Verification items for the finished model (mm, model axes). Round coordinates to 2 decimals unless told otherwise and drop trailing zeros. Order: outer loops, then holes, each group sorted by start corner. A loop starts at its lowest first (then second) coordinate and runs counter-clockwise, first axis right, second up. Notation, with made-up numbers: (23, -3) -> (68, -3) arc R14 cw to (68, 19) -> close; hole circle Ø2 at (69.5, 69). An arc over 180 degrees is marked (long way). Put each result on its own line as item: value.
```python
from build123d import *

# Parameters (mm, degrees)
PAD012_DEPTH            = 3
FILLET037_R             = 3.35
SKETCH185_R             = 1.15
POCKET053_DEPTH         = 3
POCKET056_DEPTH         = 5
SKETCH189_W             = 32
SKETCH189_H             = 20
POCKET057_DEPTH         = 1.5
BODY024_PLACEMENT_ANGLE = 149
CLONE_PLACEMENT_ANGLE   = 149


with BuildPart() as part:
    # Sketch184 → Pad012 (new body)
    with BuildSketch(Plane(origin=(0, 0, 0), x_dir=(1, 0, 0), z_dir=(0, 0, -1))):
        Polygon((101.467362, -402.500006), (130.400002, -402.500006), (135.400002, -402.500006), (135.400002, -397.500006), (174.999975, -357.90402), (174.999975, -245), (289.999995, -245), (294.999995, -245), (294.999995, -215), (289.999995, -215), (224.999995, -215), (224.999995, -199.999997), (219.999995, -199.999997), (199.999995, -199.999997), (194.999995, -199.999997), (194.999995, -215.000003), (168.459985, -215.000003), (161.999993, -198.359996), (161.999993, -115.000006), (161.999993, -110.000006), (156.999993, -110.000006), (134.576923, -122.534363), (131.999997, -126.895911), (131.999997, -200.027011), (144.989344, -239.967928), (144.989344, -343.839368), (96.467362, -392.500006), (96.467362, -397.500006), (96.467362, -402.500006), align=None)
    extrude(amount=PAD012_DEPTH)

    # Fillet037
    fillet037_edges = [part.edges().sort_by_distance(p)[0] for p in [
        (194.999995, 215.000003, -1.5),
        (168.459985, 215.000003, -1.5),
        (161.999993, 198.359996, -1.5),
        (161.999993, 110.000006, -1.5),
        (156.999993, 110.000006, -1.5),
        (134.576923, 122.534363, -1.5),
        (131.999997, 126.895911, -1.5),
        (131.999997, 200.027011, -1.5),
        (144.989344, 239.967928, -1.5),
        (144.989344, 343.839368, -1.5),
        (96.467362, 392.500006, -1.5),
        (135.400002, 397.500006, -1.5),
        (174.999975, 357.90402, -1.5),
        (174.999975, 245, -1.5),
        (294.999995, 245, -1.5),
        (294.999995, 215, -1.5),
        (224.999995, 215, -1.5),
    ]]
    fillet(fillet037_edges, radius=FILLET037_R)

    # Sketch185 (on Face5 of Fillet037) → Pocket053 (cut)
    with BuildSketch(Plane(origin=(0, 0, -3), x_dir=(1, 0, 0), z_dir=(0, 0, -1))):
        with Locations((105, -389)):
            Circle(SKETCH185_R)
        with Locations((145, -349)):
            Circle(SKETCH185_R)
        with Locations((147.500002, -309.000005)):
            Circle(SKETCH185_R)
        with Locations((147.500002, -259.000004)):
            Circle(SKETCH185_R)
        with Locations((172.500003, -259.000004)):
            Circle(SKETCH185_R)
        with Locations((172.500003, -309.000005)):
            Circle(SKETCH185_R)
        with Locations((172.500003, -349.000005)):
            Circle(SKETCH185_R)
        with Locations((147.665007, -382.765018)):
            Circle(SKETCH185_R)
        with Locations((178.000003, -242.500004)):
            Circle(SKETCH185_R)
        with Locations((218.000003, -242.500004)):
            Circle(SKETCH185_R)
        with Locations((258.000004, -242.500004)):
            Circle(SKETCH185_R)
        with Locations((258.000004, -217.500003)):
            Circle(SKETCH185_R)
        with Locations((292, -242.500004)):
            Circle(SKETCH185_R)
        with Locations((292.000004, -217.500003)):
            Circle(SKETCH185_R)
        with Locations((292.500004, -230.000003)):
            Circle(SKETCH185_R)
        with Locations((223.000003, -217.000003)):
            Circle(SKETCH185_R)
        with Locations((197, -217)):
            Circle(SKETCH185_R)
        with Locations((166.109996, -217.109995)):
            Circle(SKETCH185_R)
        with Locations((147.500002, -239)):
            Circle(SKETCH185_R)
        with Locations((141, -220)):
            Circle(SKETCH185_R)
        with Locations((134.427551, -201)):
            Circle(SKETCH185_R)
        with Locations((160.149996, -200.999996)):
            Circle(SKETCH185_R)
        with Locations((134.427551, -161)):
            Circle(SKETCH185_R)
        with Locations((159.500002, -161.000002)):
            Circle(SKETCH185_R)
        with Locations((137, -124)):
            Circle(SKETCH185_R)
        with Locations((146.849997, -118.149997)):
            Circle(SKETCH185_R)
        with Locations((159, -113)):
            Circle(SKETCH185_R)
    extrude(amount=-POCKET053_DEPTH, mode=Mode.SUBTRACT)

    # Sketch188 (on Face5 of Pocket053) → Pocket056 (cut)
    with BuildSketch(Plane(origin=(0, 0, -3), x_dir=(1, 0, 0), z_dir=(0, 0, -1))):
        Polygon((145, -269), (175, -269), (176, -269), (176, -410), (90, -410), (90, -269), align=None)
    extrude(amount=-POCKET056_DEPTH, mode=Mode.SUBTRACT)

    # Sketch189 (on Face2 of Pocket056) → Pocket057 (cut)
    with BuildSketch(Plane.XY):
        with Locations((160, 259)):
            Rectangle(SKETCH189_W, SKETCH189_H)
    extrude(amount=-POCKET057_DEPTH, mode=Mode.SUBTRACT)


with BuildPart() as part_1:
    # Body024 placement: moved
    add(part.part.moved(Location((707.641298, 2.853319, 22))).rotate(Axis((707.641298, 2.853319, 22), (0, 0, 1)), BODY024_PLACEMENT_ANGLE))


with BuildPart() as part_2:
    # Clone placement: moved
    add(part_1.part.moved(Location((477.097416, 93.907984, -22))).rotate(Axis((477.097416, 93.907984, -22), (0, 0, -1)), CLONE_PLACEMENT_ANGLE))


solid = part_2.part
```
Item 1: Release check for a two-part mould opening along X. For faces 1 (the face through (32, -14, -1.5)), 2 (the face through (17.948, -156.822, -1.479)), 3 (the face through (36.966, -66.999, -1.479)) record: pulls with the +X half, pulls with the -X half, needs draft (parallel to the pull), parting line crosses it, or undercut.
Geometry check:
face 1: needs draft
face 2: pulls with the -X half
face 3: undercut
Item 2: Material ranges on line 1 along X through (y, z) = (-76.5, -0.85); line 2 along Y through (x, z) = (105, -1.9); line 3 along X through (y, z) = (-70.5, -0.45), recorded low to high.
Geometry check:
line 1: 4 to 34
line 2: -58 to -28
line 3: 4.8 to 35.61, 67 to 97
Item 3: Sectioned sample at B-B, the plane z = -1.95. Give the number of separate pieces and of enclosed holes in the cut face, then the cut area to 3 significant figures.
Geometry check:
separate pieces: 1
enclosed holes: 21
area: 8,670 mm2
Item 4: Sectioned sample at C-C, the plane x = 110.5. Record the boundary of the cut face in (y, z).
Geometry check:
outline: (-58, -3) -> (-28, -3) -> (-28, 0) -> (-58, 0) -> close
Item 5: Sectioned sample at A-A, the plane y = -69. Record the boundary of the cut face in (x, z), then the cut area to 3 significant figures.
Geometry check:
outline: (5.29, -3) -> (36.19, -3) -> (36.19, 0) -> (5.29, 0) -> close; (67, -3) -> (97, -3) -> (97, 0) -> (67, 0) -> close
area: 183 mm2
Item 6: Depth check by flat-ended pin: pin 1 Ø2.5 at (x, y) = (19.5, -14) entering from +Z; pin 2 Ø1.5 at (x, z) = (121.5, -0.5) entering from -Y; pin 3 Ø1.5 at (y, z) = (-12.5, -1) entering from +X. Enter the tip coordinate at first touch or a pass-through.
Geometry check:
pin 1: z = -1.5
pin 2: y = -58
pin 3: x = 47
Item 7: Sectioned sample at D-D, the plane y = -107. Record the boundary of the cut face in (x, z), then the cut area to 3 significant figures.
Geometry check:
outline: (4, -3) -> (34, -3) -> (34, 0) -> (4, 0) -> close
area: 90.0 mm2
